Input: part model. Units: mm. Frame: model coordinates. A direction names the side the tool comes from. Give positions to 0.01 mm unless a question says otherwise; leave off trailing zeros. Loops run counter-clockwise (first coordinate to the right, second up) from the corner with the lowest first, then second, coordinate; pieces in that order, holes last. Notation, with made-up numbers: (-5, 45.5) - (26, 45.5) arc R22 cw to (26, 54.5) - close; hole circle Ø3 at (-5, 63). An arc over 180 degrees is marked (long way). One line per item, written item: value.
from build123d import *

# Parameters (mm, degrees)
F0_W      = 22
F0_H      = 22
F0_R      = 8
F1_DEPTH  = 1
F2_W      = 22
F2_H      = 22
F2_R      = 9.25
F3_DEPTH  = 3.5
F4_W      = 3
F4_H      = 13
F5_DEPTH  = 10
F6_W      = 10
F6_H      = 7.5
F7_DEPTH  = 3.5
F9_DEPTH  = 10
F10_DEPTH = 10


with BuildPart() as f1:
    # F0 (on Front) → F1 (new body)
    with BuildSketch(Plane.XZ):
        with Locations((11, 11)):
            Rectangle(F0_W, F0_H)
        with Locations((11, 11)):
            Circle(F0_R, mode=Mode.SUBTRACT)
    extrude(amount=F1_DEPTH)

    # F2 (on face) → F3 (join)
    with BuildSketch(Plane.XZ.offset(1)):
        with Locations((11, 11)):
            Rectangle(F2_W, F2_H)
        with Locations((11, 11)):
            Circle(F2_R, mode=Mode.SUBTRACT)
    extrude(amount=F3_DEPTH)

    # F4 (on face) → F5 (join)
    with BuildSketch(Plane(origin=(0, 0, 0), x_dir=(0, -1, 0), z_dir=(-1, 0, 0))):
        with Locations((3, 11)):
            Rectangle(F4_W, F4_H)
    extrude(amount=F5_DEPTH)

    # F6 (on face) → F7 (join)
    with BuildSketch(Plane.XZ.offset(4.5)):
        with Locations((-5, 10.75)):
            Rectangle(F6_W, F6_H)
    extrude(amount=F7_DEPTH)

    # F8 (on face) → F9 (cut)
    with BuildSketch(Plane(origin=(-10, 0, 0), x_dir=(0, -1, 0), z_dir=(-1, 0, 0))):
        Polygon((4.5, 7), (8, 7), (4.5, 8), align=None)
    extrude(amount=-F9_DEPTH, mode=Mode.SUBTRACT)

    # F8 (on face) → F10 (cut)
    with BuildSketch(Plane(origin=(-10, 0, 0), x_dir=(0, -1, 0), z_dir=(-1, 0, 0))):
        Polygon((4.5, 13.5), (8, 14.5), (4.5, 14.5), align=None)
    extrude(amount=-F10_DEPTH, mode=Mode.SUBTRACT)


solid = f1.part
Item 1: Access query for faces 4 (the face through (-5, -1.5, 11)), 5 (the face through (-5, -3, 4.5)), 6 (the face through (-5.07, -6.274, 7.493)), 7 (the face through (-5, -3, 17.5)), 8 (the face through (-5.07, -6.226, 13.993)). Directions: +Z, -Z, +X, -X, +Y, -Y. A direction counts if a zero-diameter tool reaches every point of the face in a straight line with its end or side. Return the directions, or none.
Verdict:
face 4: +Z, -Z, -X, +Y
face 5: -Z, -X, +Y, -Y
face 6: -Z, +X, -X
face 7: +Z, -X, +Y, -Y
face 8: +Z, +X, -X
Item 2: Section C-C, the plane y = -0.5. Output: boundary loops of the cut face in (x, z).
Verdict:
outline: (0, 0) - (22, 0) - (22, 22) - (0, 22) - close; hole circle Ø16 at (11, 11)
Item 3: Pin query (flat end, axial travel): P1, Ø3.5, axis at x = -7, y = -3, coming from the +Z side; P2, Ø0.9, axis at x = -3.5, y = -3.5, coming from the -Z side; P3, Ø9, axis at x = 8, z = 7, coming from the -Y side. Return the tip coordinate at first contact, or that it passes through.
Verdict:
P1: stops at z = 17.5
P2: stops at z = 4.5
P3: stops at y = -4.5
Item 4: Section B-B, the plane x = 11. Output: boundary loops of the cut face in (y, z).
Verdict:
outline: (-4.5, 0) - (0, 0) - (0, 3) - (-1, 3) - (-1, 1.75) - (-4.5, 1.75) - close; (-4.5, 20.25) - (-1, 20.25) - (-1, 19) - (0, 19) - (0, 22) - (-4.5, 22) - close
Item 5: Section D-D, the plane x = -5.5. Output: boundary loops of the cut face in (y, z), and give its area (4 significant figures).
Verdict:
outline: (-8, 7) - (-4.5, 8) - (-4.5, 4.5) - (-1.5, 4.5) - (-1.5, 17.5) - (-4.5, 17.5) - (-4.5, 13.5) - (-8, 14.5) - close
area: 61.75 mm^2
Item 6: Material intervals for L1, parallel to Z at x = 11, y = -3.25; L2, parallel to Z at x = 11, y = -0.45; L3, parallel to X at y = -3.25, z = 3.5, sorted ascending.
Verdict:
L1: z = 0 to 1.75, 20.25 to 22
L2: z = 0 to 3, 19 to 22
L3: x = 0 to 5.59, 16.41 to 22
Item 7: Draft query along Z for faces 1 (the face through (11, -2, 0)), 2 (the face through (8, -1, 19)), 3 (the face through (22, -2, 11)). Return one class per face: pulls with the +Z half, pulls with the -Z half, needs draft (parallel to the pull), parting line crosses it, or undercut.
Verdict:
face 1: pulls with the -Z half
face 2: undercut
face 3: needs draft
Item 8: Section A-A, the plane z = 11. Output: boundary loops of the cut face in (x, y).
Verdict:
outline: (-10, -8) - (0, -8) - (0, -4.5) - (1.75, -4.5) - (1.75, -1) - (3, -1) - (3, 0) - (0, 0) - (0, -1.5) - (-10, -1.5) - close; (19, -1) - (20.25, -1) - (20.25, -4.5) - (22, -4.5) - (22, 0) - (19, 0) - close
